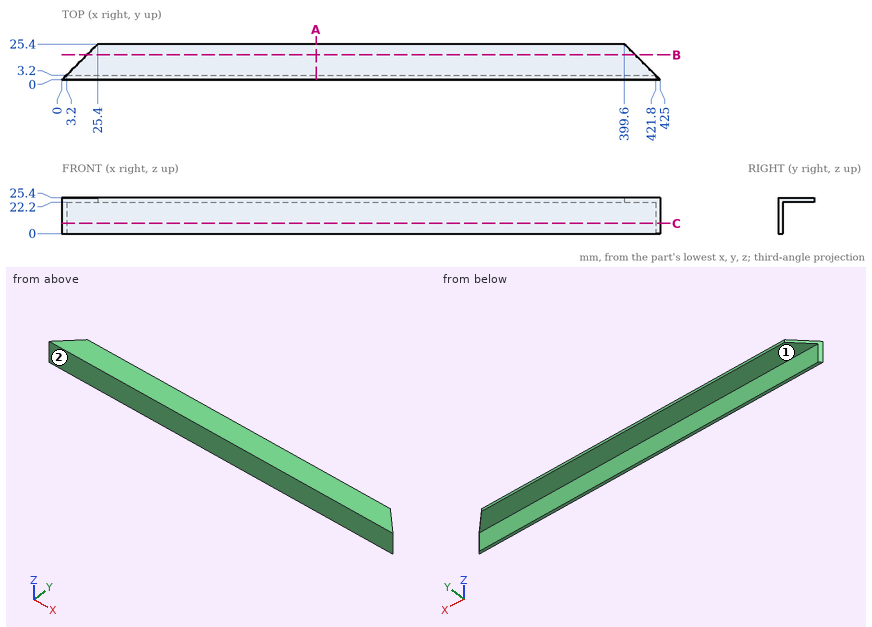
Could you check a few things on this drawing? It's one solid part, dimensions in mm from its lowest x, y, z. A direction names the side the tool comes from. Give positions to 0.01 mm unless a question says otherwise; leave off trailing zeros. Write each loop counter-clockwise with the first axis right and the second up, starting at its lowest first coordinate (ties: lowest second). Pieces come first, ordered by that corner, then holes. Notation, with made-up numbers: (29, 74) - (77, 74) arc R14 cw to (77, 92) - close; hole circle Ø7 at (33.25, 29). An arc over 180 degrees is marked (long way). Use CSV: the item, a comma, the result in double quotes. Start each with the question number.
Item 1: For the marked faces 1 and 2, which set-ups out of +Z, -Z, +X, -X, +Y, -Y let a thin tool reach every point of the face, with its end or its side?
Item 2: I want a section at C-C, the plane z = 7.25. Please give me the cut outline in (x, y), then the cut area to 3 significant figures.
Item 3: I'm going to push flat-ended pins straight in: pin 1 (1.5 mm diameter, centred on x = 123, z = 14.5, fed in from +Y); pin 2 (11 mm diameter, centred on x = 224.5, y = 11, fed in from -Z); pin 3 (8 mm diameter, centred on y = 19, z = 19, fed in from -X). Where does each tip first touch, or does it pass through?
Item 4: I want a section at B-B, the plane y = 17.75. Please give me the cut outline in (x, z).
Item 5: If I drill on line 1 along Z through (x, y) = (241, 6.25); line 2 along Y through (x, z) = (296, 20.25); line 3 along X through (y, z) = (2, 9.5), over which ranges is the centre line in solid material (lowest first)?
Item 6: I want a section at A-A, the plane x = 180.5. Please give me the cut outline in (y, z).
Findings:
1,face 1,"-Z, +X, -X, +Y"
1,face 2,"+Z, -Z, +X, -X, -Y"
2,outline,"(0, 0) - (425, 0) - (421.8, 3.2) - (3.2, 3.2) - close"
2,area,"1,350 mm2"
3,pin 1,"stops at y = 3.2"
3,pin 2,"stops at z = 22.2"
3,pin 3,"stops at x = 16.6"
4,outline,"(17.75, 22.2) - (407.25, 22.2) - (407.25, 25.4) - (17.75, 25.4) - close"
5,line 1,"z = 22.2 to 25.4"
5,line 2,"y = 0 to 3.2"
5,line 3,"x = 2 to 423"
6,outline,"(0, 0) - (3.2, 0) - (3.2, 22.2) - (25.4, 22.2) - (25.4, 25.4) - (0, 25.4) - close"
